The model under review builds one solid part; all positions refer to its coordinate system, in mm. Face numbers are marked on the shaded views. Coordinates: 2 decimals unless noted, no trailing zeros. Loops run counter-clockwise (first coordinate to the right, second up) from the corner with the lowest first, then second, coordinate; pieces in that order, holes last. Notation, with made-up numbers: M 71,55 L 99,55 A24 ccw 99,89 Z; hole C 22.5,79 d9. An arc over 180 degrees is marked long. Return JSON: item names as keys, results as strings.
```python
from build123d import *

# Parameters (mm, degrees)
F1_DEPTH   = 10.16
F4_D       = 6.35
F4_ON_F2_D = 6.35


with BuildPart() as f1:
    # F0 (on Top) → F1 (new body)
    with BuildSketch(Plane.XY):
        with BuildLine():
            Line((0, 13.7451505288), (0, 0))
            Line((0, 0), (7.1561528284, 0))
            ThreePointArc((7.1561528284, 0), (12.2831791104, 2.1876687498), (17.4102053924, 0))
            Line((17.4102053924, 0), (24.2389943451, 0))
            Line((24.2389943451, 0), (24.2389943451, 13.7451505288))
            Line((24.2389943451, 13.7451505288), (17.0903896092, 13.7451505288))
            ThreePointArc((17.0903896092, 13.7451505288), (12.240587268, 11.4840131173), (7.3907849269, 13.7451505288))
            Line((7.3907849269, 13.7451505288), (0, 13.7451505288))
        make_face()
    extrude(amount=F1_DEPTH)

    # F4 (through all)
    with Locations(Plane.YZ.offset(24.2389943451)):
        with Locations((4.0866504423, 8.0641144887)):
            Hole(F4_D / 2)

    # F4 on F2 (through all)
    with Locations(Plane(origin=(0, 0, 0), x_dir=(0, -1, 0), z_dir=(-1, 0, 0))):
        with Locations((-6.9927107543, 4.7133392654)):
            Hole(F4_ON_F2_D / 2)


solid = f1.part
```
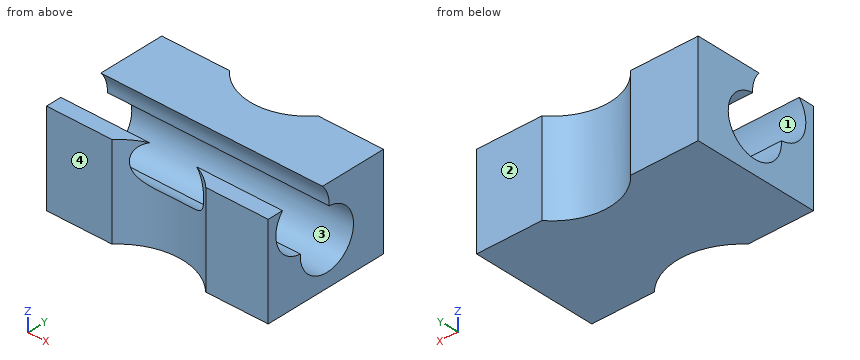
1. To check wall thickness, follow line 1 (Y direction, x = 3.75, z = 4.75); line 2 (Y direction, x = 12, z = 2.25); line 3 (Z direction, x = 10.5, y = 8). State the ranges of each line that lie inside material, in increasing order.
Check values:
{"line 1": "0 to 3.82, 10.17 to 13.75", "line 2": "2.18 to 4.99, 9 to 11.49", "line 3": "0 to 1.7, 7.72 to 10.16"}
2. Add section B-B on y = 12. Give the boundary of the cut face in (x, z), plus the area to 3 significant figures.
Check values:
{"outline": "M 0,0 L 9.74,0 L 9.74,10.16 L 0,10.16 Z; M 14.74,0 L 24.24,0 L 24.24,10.16 L 14.74,10.16 Z", "area": "195 mm²"}
3. The part is to be moulded in two halves that separate along Y. For the marked faces 1, 2, 3 and 4, say which applies: released by +Y, released by -Y, zero draft, split by the parting line, or undercut.
Check values:
{"face 1": "undercut", "face 2": "released by +Y", "face 3": "undercut", "face 4": "released by -Y"}
4. Add section C-C on z = 7.5. Give the boundary of the cut face in (x, y).
Check values:
{"outline": "M 0,0 L 7.16,0 A7.1 cw 8.3,0.96 L 0,0.96 Z; M 0,8.51 L 24.24,8.51 L 24.24,13.75 L 17.09,13.75 A6.33 cw 7.39,13.75 L 0,13.75 Z; M 16.27,0.96 A7.1 cw 17.41,0 L 24.24,0 L 24.24,0.96 Z"}
5. Add section D-D on z = 3. Give the boundary of the cut face in (x, y), plus the area to 3 significant figures.
Check values:
{"outline": "M 0,0 L 7.16,0 A7.1 cw 17.41,0 L 24.24,0 L 24.24,4.32 L 0,4.32 Z; M 0,9.67 L 24.24,9.67 L 24.24,13.75 L 17.09,13.75 A6.33 cw 7.39,13.75 L 0,13.75 Z", "area": "173 mm²"}
6. Add section A-A on z = 1. Give the boundary of the cut face in (x, y).
Check values:
{"outline": "M 0,0 L 7.16,0 A7.1 cw 17.41,0 L 24.24,0 L 24.24,13.75 L 17.09,13.75 A6.33 cw 7.39,13.75 L 0,13.75 Z"}
